Input: part model. Units: mm. Frame: model coordinates. A direction names the side the tool comes from. Round coordinates to 2 decimals unless told otherwise and drop trailing zeros. Loops run counter-clockwise (first coordinate to the right, second up) from the corner with the lowest first, then second, coordinate; pieces in that order, holes last.
(1) Line query: line 1 (Y direction, x = 0, z = 2.4); line 2 (Y direction, x = 13.5, z = 2); line 3 (Y direction, x = 26, z = 1.75). Output: solid intervals per line, ascending.
(2) First-contact query: pin 1 Ø2 at (x, z) = (-39, -2) entering from -Y; pin 2 Ø12 at (x, y) = (4.5, -29.5) entering from -Z; pin 3 Ø0.6 at (x, z) = (-38.5, -2.5) entering from +Y. Flat tips, straight axial feed; report the tip coordinate or a pass-through.
(3) Cut plane D-D, the plane y = -7. Output: boundary loops of the cut face in (x, z), and give its area (3 significant figures).
(4) Access query for faces 1 (the face through (-39, 28.5, -4)), 2 (the face through (-38, -33, -4)), 3 (the face through (39, 33, -8)), 4 (the face through (27.5, 41, 1)). Directions: +Z, -Z, +X, -X, +Y, -Y. A direction counts if a zero-diameter tool reaches every point of the face in a straight line with its end or side. Return the directions, or none.
(5) Cut plane B-B, the plane z = -2.25. Output: boundary loops of the cut face in (x, y), and give its area (3 significant figures).
(6) Cut plane A-A, the plane y = -30. Output: boundary loops of the cut face in (x, z), and give its area (3 significant figures).
(7) Cut plane C-C, the plane x = 0. Output: boundary loops of the cut face in (y, z), and give its area (3 significant figures).
from build123d import *

# Parameters (mm, degrees)
SKETCH1_W           = 80
SKETCH1_H           = 100
SKETCH1_R           = 12.5
SKETCH1_W_2         = 55
SKETCH1_H_2         = 11.012232525
BOSS_EXTRUDE4_DEPTH = 3
SKETCH4_W           = 2
SKETCH4_H           = 8
BOSS_EXTRUDE7_DEPTH = 8


with BuildPart() as part:
    # Sketch1 → Boss-Extrude4 (new body)
    with BuildSketch(Plane.XY):
        Rectangle(SKETCH1_W, SKETCH1_H)
        Circle(SKETCH1_R, mode=Mode.SUBTRACT)
        with BuildLine():
            Line((-27.5, 32.5), (27.5, 32.5))
            Line((27.5, 32.5), (9.624571705, 14.615663498))
            ThreePointArc((9.624571705, 14.615663498), (0.00658569, 17.499998761), (-9.613568497, 14.622903294))
            Line((-9.613568497, 14.622903294), (-27.5, 32.5))
        make_face(mode=Mode.SUBTRACT)
        with BuildLine():
            Line((-32.5, 27.5), (-32.5, -27.529900959))
            Line((-32.5, -27.529900959), (-14.610866481, -9.631852402))
            ThreePointArc((-14.610866481, -9.631852402), (-17.49999836, -0.007575188), (-14.619199644, 9.619199644))
            Line((-14.619199644, 9.619199644), (-32.5, 27.5))
        make_face(mode=Mode.SUBTRACT)
        with BuildLine():
            Line((-27.5, -32.5), (27.5, -32.5))
            Line((27.5, -32.5), (9.619199644, -14.619199644))
            ThreePointArc((9.619199644, -14.619199644), (0, -17.5), (-9.619199644, -14.619199644))
            Line((-9.619199644, -14.619199644), (-27.5, -32.5))
        make_face(mode=Mode.SUBTRACT)
        with BuildLine():
            Line((32.5, 27.5), (14.619199644, 9.619199644))
            ThreePointArc((14.619199644, 9.619199644), (17.4999982, 0.007937724), (14.627919862, -9.60593361))
            Line((14.627919862, -9.60593361), (32.5, -27.5))
            Line((32.5, -27.5), (32.5, 27.5))
        make_face(mode=Mode.SUBTRACT)
        with Locations((0, -41.233086376)):
            Rectangle(SKETCH1_W_2, SKETCH1_H_2, mode=Mode.SUBTRACT)
        with Locations((0, 41.233086376)):
            Rectangle(SKETCH1_W_2, SKETCH1_H_2, mode=Mode.SUBTRACT)
    extrude(amount=BOSS_EXTRUDE4_DEPTH)

    # Sketch4 → Boss-Extrude7 (add)
    with BuildSketch(Plane(origin=(0, 0, 0), x_dir=(-1, 0, 0), z_dir=(0, 0, -1))):
        with Locations((-39, 32.5)):
            Rectangle(SKETCH4_W, SKETCH4_H)
        with Locations((-39, -32.5)):
            Rectangle(SKETCH4_W, SKETCH4_H)
        with Locations((39, 32.5)):
            Rectangle(SKETCH4_W, SKETCH4_H)
        with Locations((39, -32.5)):
            Rectangle(SKETCH4_W, SKETCH4_H)
    extrude(amount=BOSS_EXTRUDE7_DEPTH)


solid = part.part
Reported:
1. line 1: y = -50 to -46.74, -35.73 to -32.5, -17.5 to -12.5, 12.5 to 17.5, 32.5 to 35.73, 46.74 to 50
1. line 2: y = -50 to -46.74, -35.73 to -32.5, -18.5 to 18.49, 32.5 to 35.73, 46.74 to 50
1. line 3: y = -50 to -46.74, -35.73 to -32.5, -31 to -20.99, 21 to 31, 32.5 to 35.73, 46.74 to 50
2. pin 1: stops at y = -36.5
2. pin 2: stops at z = 0
2. pin 3: stops at y = 36.5
3. outline: (-40, 0) - (-32.5, 0) - (-32.5, 3) - (-40, 3) - close; (-16.04, 0) - (-10.36, 0) - (-10.36, 3) - (-16.04, 3) - close; (10.36, 0) - (16.04, 0) - (16.04, 3) - (10.36, 3) - close; (32.5, 0) - (40, 0) - (40, 3) - (32.5, 3) - close
3. area: 79.1 mm2
4. face 1: -Z, +X, -X
4. face 2: -Z, +Y, -Y
4. face 3: -Z, +X, -X, +Y, -Y
4. face 4: +Z, -Z
5. outline: (-40, -36.5) - (-38, -36.5) - (-38, -28.5) - (-40, -28.5) - close; (-40, 28.5) - (-38, 28.5) - (-38, 36.5) - (-40, 36.5) - close; (38, -36.5) - (40, -36.5) - (40, -28.5) - (38, -28.5) - close; (38, 28.5) - (40, 28.5) - (40, 36.5) - (38, 36.5) - close
5. area: 64.0 mm2
6. outline: (-40, -8) - (-38, -8) - (-38, 0) - (-25, 0) - (-25, 3) - (-40, 3) - close; (25, 0) - (38, 0) - (38, -8) - (40, -8) - (40, 3) - (25, 3) - close
6. area: 122 mm2
7. outline: (-50, 0) - (-46.74, 0) - (-46.74, 3) - (-50, 3) - close; (-35.73, 0) - (-32.5, 0) - (-32.5, 3) - (-35.73, 3) - close; (-17.5, 0) - (-12.5, 0) - (-12.5, 3) - (-17.5, 3) - close; (12.5, 0) - (17.5, 0) - (17.5, 3) - (12.5, 3) - close; (32.5, 0) - (35.73, 0) - (35.73, 3) - (32.5, 3) - close; (46.74, 0) - (50, 0) - (50, 3) - (46.74, 3) - close
7. area: 68.9 mm2
